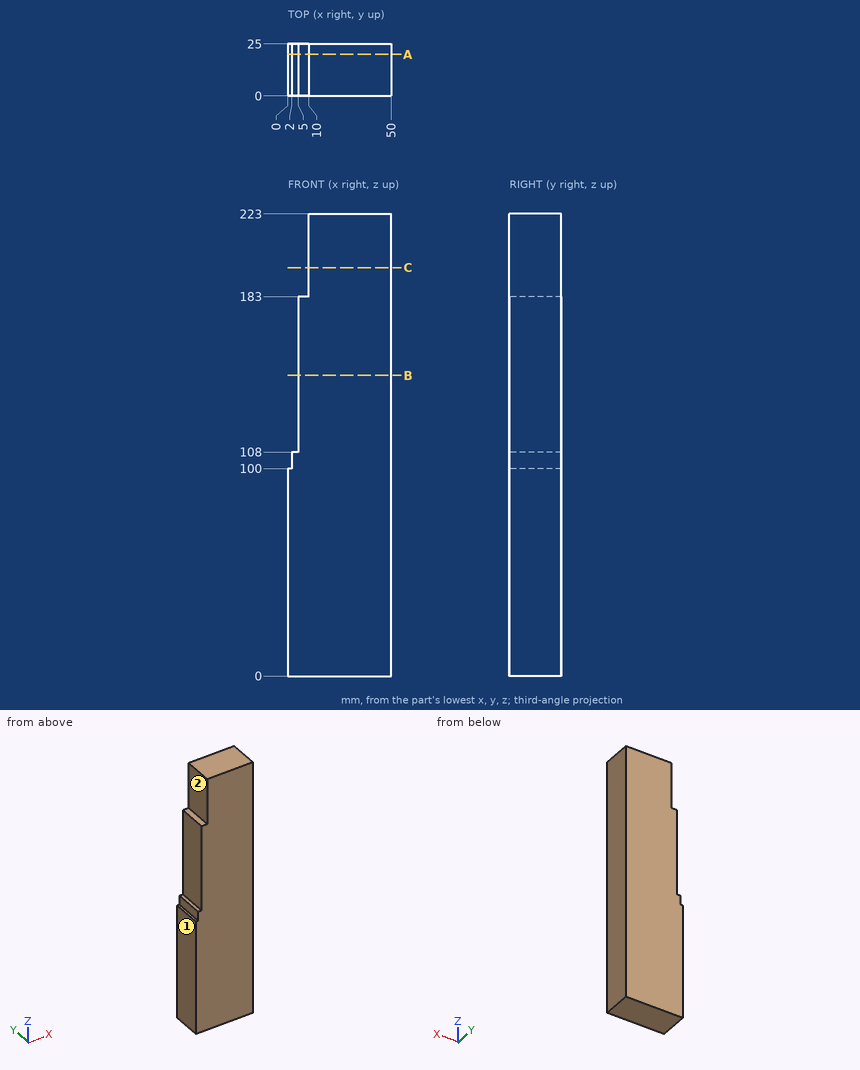
Geometry check sheet. Reference: drawing and pictorial views, mm from the part's lowest x, y, z. A direction names the side the tool comes from. Round coordinates to 2 decimals unless told otherwise and drop trailing zeros. Loops run counter-clockwise (first coordinate to the right, second up) from the corner with the lowest first, then second, coordinate; pieces in that order, holes last. Notation, with made-up numbers: (34.25, 10.25) - (71.25, 10.25) arc R14 ccw to (71.25, 22.25) - close; hole circle Ø3 at (45.5, 33.25). An arc over 180 degrees is marked (long way). Answer as CSV lines item,"result".
(1) Set-up check for the marked faces 1 and 2: record each of +Z, -Z, +X, -X, +Y, -Y from which the full face is reachable in a straight line by a thin tool's end or side.
Output values:
face 1,"+Z, -Z, -X, +Y, -Y"
face 2,"+Z, -X, +Y, -Y"
(2) Cross-section at C-C, the plane z = 197. Enter the section's corners in (x, y).
Output values:
outline,"(10, 0) - (50, 0) - (50, 25) - (10, 25) - close"
(3) Cross-section at B-B, the plane z = 145. Enter the section's corners in (x, y).
Output values:
outline,"(5, 0) - (50, 0) - (50, 25) - (5, 25) - close"
(4) Cross-section at A-A, the plane y = 20. Enter the section's corners in (x, z).
Output values:
outline,"(0, 0) - (50, 0) - (50, 223) - (10, 223) - (10, 183) - (5, 183) - (5, 108) - (2, 108) - (2, 100) - (0, 100) - close"
(5) Depth check by flat-ended pin: pin 1 Ø1.5 at (x, y) = (4, 18) entering from +Z; pin 2 Ø2 at (y, z) = (3, 102.5) entering from -X; pin 3 Ø0.6 at (x, y) = (1, 13.5) entering from +Z. Enter the tip coordinate at first touch or a pass-through.
Output values:
pin 1,"stops at z = 108"
pin 2,"stops at x = 2"
pin 3,"stops at z = 100"
(6) Material ranges on line 1 along X through (y, z) = (6.75, 155); line 2 along Z through (x, y) = (3.5, 9); line 3 along X through (y, z) = (3, 195.5), recorded low to high.
Output values:
line 1,"x = 5 to 50"
line 2,"z = 0 to 108"
line 3,"x = 10 to 50"
